Can you work these out from the model? Positions are in its coordinate system, mm. A direction names the side the tool comes from. Give positions to 0.01 mm unless a question says otherwise; leave off trailing zeros. Order: outer loops, then holes, each group sorted by start corner. A loop starts at its lowest first (then second) coordinate and runs counter-clockwise, first axis right, second up. Notation, with made-up numbers: (-26.5, -5.5) - (-15.5, -5.5) arc R21 cw to (-15.5, 33.5) - close; hole circle Ø2 at (30.25, -19). An arc over 180 degrees is marked (long way). Answer as CSV lines item,"result".
```python
from build123d import *

# Parameters (mm, degrees)
SKETCH2_R           = 3.95
BOSS_EXTRUDE1_DEPTH = 3.25
SKETCH5_R           = 3.5
BOSS_EXTRUDE4_DEPTH = 2
SKETCH7_R           = 5.45
BOSS_EXTRUDE5_DEPTH = 1
CUT_EXTRUDE1_DEPTH  = 8.1


with BuildPart() as part:
    # Sketch2 → Boss-Extrude1 (new, symmetric)
    with BuildSketch(Plane(origin=(0, 0, 0), x_dir=(1, 0, 0), z_dir=(0, 1, 0))):
        with Locations(Location((0, 0, 0), (0, 0, 90))):
            Circle(SKETCH2_R)
    extrude(amount=BOSS_EXTRUDE1_DEPTH, both=True)

    # Sketch5 → Boss-Extrude4 (add)
    with BuildSketch(Plane.XZ.offset(3.25)):
        with Locations(Location((0, 0, 0), (0, 0, 90))):
            Circle(SKETCH5_R)
    extrude(amount=BOSS_EXTRUDE4_DEPTH)

    # Sketch7 → Boss-Extrude5 (add)
    with BuildSketch(Plane.XZ.offset(3.25)):
        with Locations(Location((0, 0, 0), (0, 0, 270))):
            Circle(SKETCH7_R)
    extrude(amount=BOSS_EXTRUDE5_DEPTH)

    # Sketch6 → Cut-Extrude1 (cut)
    with BuildSketch(Plane.XZ.offset(5.25)):
        with BuildLine():
            ThreePointArc((2.075, 0), (-0.799143979, 1.91493966), (-1.459451952, -1.475))
            Line((-1.459451952, -1.475), (1.459451952, -1.475))
            ThreePointArc((1.459451952, -1.475), (1.91493966, -0.799143979), (2.075, 0))
        make_face()
    extrude(amount=-CUT_EXTRUDE1_DEPTH, mode=Mode.SUBTRACT)


solid = part.part
```
1) Which directions (+Z, -Z, +X, -X, +Y, -Y) give clear straight access to the entire face, cutting with the end or side of a thin tool? Please do faces 4 (the cylindrical face through (3.417, -4.743, -0.759)), 5 (the flat face through (0, 3.25, 0)), 6 (the cylindrical face through (-2.67, 0.05, 2.91)).
Answer block:
face 4,"-Y"
face 5,"+Z, -Z, +X, -X, +Y"
face 6,"+Y"
2) If we mould it in two halves opening along Z, with no side actions, what happens to faces 1 (the flat face through (0, -5.25, -2)), 2 (the flat face through (0, -1, -1.475)), 3 (the cylindrical face through (-5.32, -3.74, 1.18))? For each: +Z half, -Z half, draft (parallel to the pull), parting line (faces both ways), or undercut.
Answer block:
face 1,"draft"
face 2,"undercut"
face 3,"parting line"
3) I want a section at D-D on y = -4. Write out the boundary of the cut face in (x, z) (3 decimals), plus the area to 3 significant figures.
Answer block:
outline,"circle Ø10.9 at (0, 0); hole (-1.459, -1.475) - (1.459, -1.475) arc R2.075 ccw (long way) to start"
area,"81.0 mm2"
4) I want a section at A-A on y = -2.75. Write out the boundary of the cut face in (x, z) (3 decimals).
Answer block:
outline,"circle Ø7.9 at (0, 0); hole (-1.459, -1.475) - (1.459, -1.475) arc R2.075 ccw (long way) to start"
5) I'm going to push flat-ended pins straight in: P1, Ø3, axis at x = 1.5, y = -0.5, coming from the +Z side; P2, Ø3.5, axis at x = 0, z = 0, coming from the -Y side; P3, Ø1.1, axis at x = 0, z = 0, coming from the -Y side; P4, Ø3, axis at y = 0.5, z = 3, coming from the +X side. Where does each tip first touch, or does it pass through?
Answer block:
P1,"z = 3.95"
P2,"y = -5.25"
P3,"y = 2.85"
P4,"x = 3.65"
6) I want a section at B-B on x = -0.5. Write out the boundary of the cut face in (y, z) (3 decimals), plus the area to 3 significant figures.
Answer block:
outline,"(-5.25, -3.464) - (-4.25, -3.464) - (-4.25, -5.427) - (-3.25, -5.427) - (-3.25, -3.918) - (3.25, -3.918) - (3.25, 3.918) - (-3.25, 3.918) - (-3.25, 5.427) - (-4.25, 5.427) - (-4.25, 3.464) - (-5.25, 3.464) - (-5.25, 2.014) - (2.85, 2.014) - (2.85, -1.475) - (-5.25, -1.475) - close"
area,"40.5 mm2"
7) I need wall thicknesses on line 1 along X through (y, z) = (-1.75, 0) (3 decimals); line 2 along X through (y, z) = (0.5, 1); line 3 along Y through (x, z) = (-1.5, 4.5). Which ranges of each line are inside material? Lowest first, please. Write a range as [from, to].
Answer block:
line 1,"[-3.95, -2.075], [2.075, 3.95]"
line 2,"[-3.82, -1.82], [1.82, 3.82]"
line 3,"[-4.25, -3.25]"
8) I want a section at C-C on z = -0.75. Write out the boundary of the cut face in (x, y), plus the area to 3 significant figures.
Answer block:
outline,"(-5.4, -4.25) - (-3.42, -4.25) - (-3.42, -5.25) - (-1.93, -5.25) - (-1.93, 2.85) - (1.93, 2.85) - (1.93, -5.25) - (3.42, -5.25) - (3.42, -4.25) - (5.4, -4.25) - (5.4, -3.25) - (3.88, -3.25) - (3.88, 3.25) - (-3.88, 3.25) - (-3.88, -3.25) - (-5.4, -3.25) - close"
area,"36.7 mm2"
